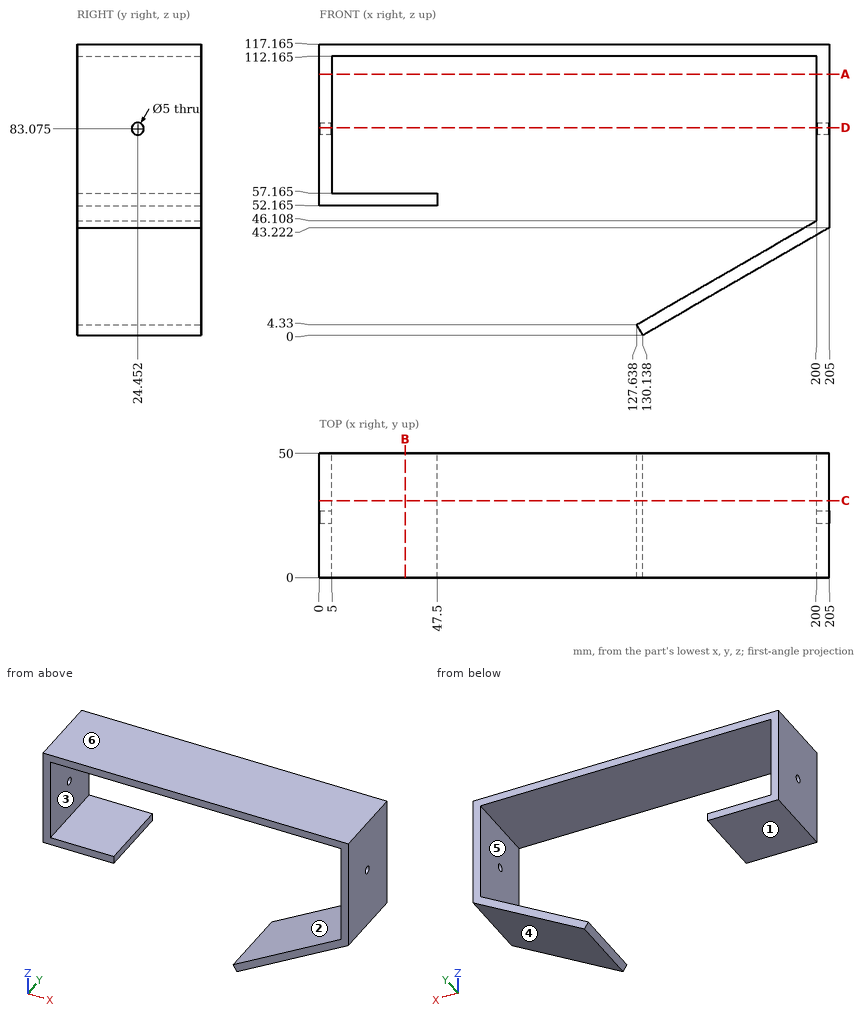
Print and shaded views of the part. All mm, measured from the part's lowest x, y and z. A direction names the side the tool comes from. Round coordinates to 2 decimals unless told otherwise and drop trailing zeros. Loops run counter-clockwise (first coordinate to the right, second up) from the corner with the lowest first, then second, coordinate; pieces in that order, holes last. Notation, with made-up numbers: (-20.5, -11) -> (1.5, -11) arc R28 ccw to (1.5, 18) -> close; hole circle Ø6 at (31.25, 24.25). An arc over 180 degrees is marked (long way). Use CSV: the item, a comma, the result in double quotes. Start each with the question number.
1) Cut at B-B, the plane x = 34.5. Write the cut outline in (y, z) (1 decimal).
2) Cut at D-D, the plane z = 83.5. Write the cut outline in (x, y) (1 decimal).
3) Which spindle directions (+Z, -Z, +X, -X, +Y, -Y) get a long thin tool onto all of the face, cutting with end or side? Do the marked faces 1, 2 and 3. Say none if no direction does.
4) Wall check: L1, parallel to X at y = 18, z = 102; L2, parallel to Z at x = 35.5, y = 28.5 (1 decimal); L3, parallel to Z at x = 51.5, y = 45 (1 decimal). Give the ranges that are in metal, low to high. Write a range as [from, to].
5) Pull direction Z, two halves, no side cores. Call the marked faces 4, 5 and 6: +Z half, -Z half, draft (parallel to the pull), parting line (faces both ways), or undercut.
6) Cut at A-A, the plane z = 105. Write the cut outline in (x, y).
7) Drop flat-ended pins along their axis: P1, Ø1, axis at x = 79.5, y = 32.5, coming from the -Z side (1 decimal); P2, Ø8, axis at x = 22, y = 14.5, coming from the -Z side (1 decimal); P3, Ø8, axis at y = 10, z = 14, coming from the +X side (1 decimal). Give the stop position or say it passes through.
8) Cut at C-C, the plane y = 31. Write the cut outline in (x, z) (1 decimal), plus the area to 3 significant figures.
Determined:
1,outline,"(0, 52.2) -> (50, 52.2) -> (50, 57.2) -> (0, 57.2) -> close; (0, 112.2) -> (50, 112.2) -> (50, 117.2) -> (0, 117.2) -> close"
2,outline,"(0, 0) -> (5, 0) -> (5, 22) -> (0, 22) -> close; (0, 26.9) -> (5, 26.9) -> (5, 50) -> (0, 50) -> close; (200, 0) -> (205, 0) -> (205, 22) -> (200, 22) -> close; (200, 26.9) -> (205, 26.9) -> (205, 50) -> (200, 50) -> close"
3,face 1,"-Z, -X, +Y, -Y"
3,face 2,"-X, +Y, -Y"
3,face 3,"+Y, -Y"
4,L1,"x = [0, 5], [200, 205]"
4,L2,"z = [52.2, 57.2], [112.2, 117.2]"
4,L3,"z = [112.2, 117.2]"
5,face 4,"-Z half"
5,face 5,"undercut"
5,face 6,"+Z half"
6,outline,"(0, 0) -> (5, 0) -> (5, 50) -> (0, 50) -> close; (200, 0) -> (205, 0) -> (205, 50) -> (200, 50) -> close"
7,P1,"stops at z = 112.2"
7,P2,"stops at z = 52.2"
7,P3,"stops at x = 161.3"
8,outline,"(0, 52.2) -> (47.5, 52.2) -> (47.5, 57.2) -> (5, 57.2) -> (5, 112.2) -> (200, 112.2) -> (200, 46.1) -> (127.6, 4.3) -> (130.1, 0) -> (205, 43.2) -> (205, 117.2) -> (0, 117.2) -> close"
8,area,"2,300 mm2"
